```python
from build123d import *

# Parameters (mm, degrees)
F0_W      = 60
F0_H      = 26
F1_DEPTH  = 40
F5_R      = 2
F6_DEPTH  = 13
F8_D      = 3.3
F8_DEPTH  = 9
F8_TIP    = 0.9914200214
F9_R      = 4.3298566402
F10_DEPTH = 6
F11_W     = 20
F11_H     = 26
F12_DEPTH = 25
F13_R     = 2


with BuildPart() as f1:
    # F0 (on Top) → F1 (new body)
    with BuildSketch(Plane.XY):
        with Locations((30, 13)):
            Rectangle(F0_W, F0_H)
    extrude(amount=F1_DEPTH)

    # F3 (on offset) → F4 (revolve, cut)
    with BuildSketch(Plane.XZ.offset(-15)):
        with BuildLine():
            Line((35, 40), (30, 40))
            Line((30, 40), (30, 5))
            Line((30, 5), (32, 5))
            Line((32, 5), (32, 34.1348334202))
            ThreePointArc((32, 34.1348334202), (32.2309171832, 35.6367818503), (32.9023396346, 37))
            Line((32.9023396346, 37), (35, 40))
        make_face()
    revolve(axis=Axis((30, 15, 22.5), (0, 0, -1)), mode=Mode.SUBTRACT)

    # F5 (on face) → F6 (cut)
    with BuildSketch(Plane(origin=(0, 26, 0), x_dir=(-1, 0, 0), z_dir=(0, 1, 0))):
        with Locations((-30, 7)):
            Circle(F5_R)
    extrude(amount=-F6_DEPTH, mode=Mode.SUBTRACT)

    # F8
    with Locations(Plane.XY.offset(40)):
        with Locations((8, 15), (52, 15)):
            Hole(F8_D / 2, depth=F8_DEPTH)
            with Locations((0, 0, -(F8_DEPTH + F8_TIP / 2))):  # 118° drill point
                Cone(0, F8_D / 2, F8_TIP, mode=Mode.SUBTRACT)

    # F9 (on face) → F10 (cut)
    with BuildSketch(Plane(origin=(0, 26, 0), x_dir=(-1, 0, 0), z_dir=(0, 1, 0))):
        with Locations((-30, 7)):
            Circle(F9_R)
    extrude(amount=-F10_DEPTH, mode=Mode.SUBTRACT)

    # F11 (on face) → F12 (cut)
    with BuildSketch(Plane(origin=(0, 0, 0), x_dir=(1, 0, 0), z_dir=(0, 0, -1))):
        with Locations((10, -13)):
            Rectangle(F11_W, F11_H)
        with Locations((50, -13)):
            Rectangle(F11_W, F11_H)
    extrude(amount=-F12_DEPTH, mode=Mode.SUBTRACT)

    # F13
    f13_edges = [f1.edges().sort_by_distance(p)[0] for p in [
        (30, 26, 40),
        (30, 0, 40),
        (60, 13, 40),
        (0, 13, 40),
        (0, 0, 32.5),
        (10, 0, 25),
        (0, 13, 25),
        (20, 0, 12.5),
        (20, 13, 25),
        (20, 26, 12.5),
        (20, 13, 0),
        (30, 26, 0),
        (30, 0, 0),
        (40, 13, 0),
        (40, 26, 12.5),
        (40, 13, 25),
        (50, 26, 25),
        (60, 13, 25),
        (50, 0, 25),
        (40, 0, 12.5),
        (60, 26, 32.5),
        (60, 0, 32.5),
        (0, 26, 32.5),
        (10, 26, 25),
    ]]
    fillet(f13_edges, radius=F13_R)


solid = f1.part
```
Geometry check sheet. Reference: the model listing, model coordinates, mm. A direction names the side the tool comes from. Give positions to 0.01 mm unless a question says otherwise; leave off trailing zeros. Order: outer loops, then holes, each group sorted by start corner. A loop starts at its lowest first (then second) coordinate and runs counter-clockwise, first axis right, second up. Notation, with made-up numbers: (23, 57) - (64, 57) arc R20 cw to (64, 93) - close; hole circle Ø5 at (-36.5, 22.5). An arc over 180 degrees is marked (long way). Answer in a Markdown table with one row per item. Add a question column.
Q1. Cross-section at D-D, the plane z = 4. Enter the section's corners in (x, y), then the cut area to 3 significant figures.
Q2. Mould release check, pull along X, two halves, no side actions. Record for faces 4 (the cylindrical face through (28, 15, 6)), 5 (the flat face through (40, 13, 12)), 6 (the cylindrical face through (10.11, 0.6, 25.57)): pulls with the +X half, pulls with the -X half, needs draft (parallel to the pull), parting line crosses it, or undercut.
Q3. Cross-section at A-A, the plane z = 18. Enter the section's corners in (x, y), then the cut area to 3 significant figures.
Q4. Cross-section at C-C, the plane x = 16.5. Enter the section's corners in (y, z), then the cut area to 3 significant figures.
Q5. Tool access check on faces 1 (the cylindrical face through (32, 15, 6)), 2 (the flat face through (10, 13, 25)), 3 (the cylindrical face through (32, 14, 7)). Record the directions out of +Z, -Z, +X, -X, +Y, -Y that give a thin tool (end or side, any length) a straight path to the whole face; none if there is none.
Q6. Material ranges on probe 1 along X at (y, z) = (15, 33.75); probe 2 along Y at (x, z) = (52, 34); probe 3 along X at (y, z) = (15, 35.5), recorded low to high. Write a range as from..to.
Q7. Cross-section at B-B, the plane y = 7.5. Enter the section's corners in (x, z), then the cut area to 3 significant figures.
Q8. Gauge pin test, flat ends, axial feed: pin 1 (2.5 mm diameter, centred on x = 28, z = 8, fed in from +Y); pin 2 (2 mm diameter, centred on y = 13.5, z = 11.5, fed in from -X); pin 3 (6.5 mm diameter, centred on x = 30, y = 15, fed in from +Z). Record the tip position at first contact, or that the pin passes through.
Check values:
| question | item | result |
|---|---|---|
| 1 | outline | (20, 2) arc R2 ccw to (22, 0) - (38, 0) arc R2 ccw to (40, 2) - (40, 24) arc R2 ccw to (38, 26) - (33.12, 26) - (33.12, 20) - (26.88, 20) - (26.88, 26) - (22, 26) arc R2 ccw to (20, 24) - close |
| 1 | area | 479 mm^2 |
| 2 | face 4 | undercut |
| 2 | face 5 | pulls with the +X half |
| 2 | face 6 | needs draft |
| 3 | outline | (20, 2) arc R2 ccw to (22, 0) - (38, 0) arc R2 ccw to (40, 2) - (40, 24) arc R2 ccw to (38, 26) - (22, 26) arc R2 ccw to (20, 24) - close; hole circle Ø4 at (30, 15) |
| 3 | area | 504 mm^2 |
| 4 | outline | (0, 27) arc R2 ccw to (2, 25) - (24, 25) arc R2 ccw to (26, 27) - (26, 38) arc R2 ccw to (24, 40) - (2, 40) arc R2 ccw to (0, 38) - close |
| 4 | area | 387 mm^2 |
| 5 | face 1 | +Z |
| 5 | face 2 | -Z, -X, +Y, -Y |
| 5 | face 3 | +Y |
| 6 | probe 1 | x = 0..6.35, 9.65..28, 32..50.35, 53.65..60 |
| 6 | probe 2 | y = 0..13.35, 16.65..26 |
| 6 | probe 3 | x = 0..6.35, 9.65..27.81, 32.19..50.35, 53.65..60 |
| 7 | outline | (0, 27) arc R2 ccw to (2, 25) - (18, 25) arc R2 cw to (20, 23) - (20, 2) arc R2 ccw to (22, 0) - (38, 0) arc R2 ccw to (40, 2) - (40, 23) arc R2 cw to (42, 25) - (58, 25) arc R2 ccw to (60, 27) - (60, 38) arc R2 ccw to (58, 40) - (2, 40) arc R2 ccw to (0, 38) - close |
| 7 | area | 1,400 mm^2 |
| 8 | pin 1 | stops at y = 20 |
| 8 | pin 2 | stops at x = 20 |
| 8 | pin 3 | stops at z = 37.5 |
